```python
from build123d import *

# Parameters (mm, degrees)
SKETCH1_R           = 15
SKETCH1_R_2         = 3
BOSS_EXTRUDE1_DEPTH = 4
SKETCH2_R           = 15
SKETCH2_R_2         = 13
EXTRUDE_THIN1_DEPTH = 10
SKETCH3_R           = 25
SKETCH3_R_2         = 13
BOSS_EXTRUDE2_DEPTH = 4
CUT_EXTRUDE1_REACH  = 20
SKETCH4_R           = 1.75


with BuildPart() as part:
    # Sketch1 → Boss-Extrude1 (new body)
    with BuildSketch(Plane(origin=(0, 0, 0), x_dir=(1, 0, 0), z_dir=(0, 1, 0))):
        Circle(SKETCH1_R)
        Circle(SKETCH1_R_2, mode=Mode.SUBTRACT)
    extrude(amount=BOSS_EXTRUDE1_DEPTH)

    # Sketch2 → Extrude-Thin1 (add)
    with BuildSketch(Plane(origin=(0, 4, 0), x_dir=(1, 0, 0), z_dir=(0, 1, 0))):
        Circle(SKETCH2_R)
        Circle(SKETCH2_R_2, mode=Mode.SUBTRACT)
    extrude(amount=EXTRUDE_THIN1_DEPTH)

    # Sketch3 → Boss-Extrude2 (add)
    with BuildSketch(Plane(origin=(0, 14, 0), x_dir=(1, 0, 0), z_dir=(0, 1, 0))):
        Circle(SKETCH3_R)
        Circle(SKETCH3_R_2, mode=Mode.SUBTRACT)
    extrude(amount=BOSS_EXTRUDE2_DEPTH)

    # Sketch4 → Cut-Extrude1 (cut, up to next)
    with BuildSketch(Plane(origin=(0, 18, 0), x_dir=(1, 0, 0), z_dir=(0, 1, 0)), mode=Mode.PRIVATE) as cut_extrude1_sk1:
        with Locations((-17.320508076, 10)):
            Circle(SKETCH4_R)
    cut_extrude1_tool1 = extrude(cut_extrude1_sk1.sketch, amount=-CUT_EXTRUDE1_REACH, mode=Mode.PRIVATE) & part.part
    add(cut_extrude1_tool1.solids().sort_by_distance((-17.320508, 18, -10))[0], mode=Mode.SUBTRACT)
    # Sketch4 → Cut-Extrude1 (cut, up to next)
    with BuildSketch(Plane(origin=(0, 18, 0), x_dir=(1, 0, 0), z_dir=(0, 1, 0)), mode=Mode.PRIVATE) as cut_extrude1_sk2:
        with Locations((17.320508076, 10)):
            Circle(SKETCH4_R)
    cut_extrude1_tool2 = extrude(cut_extrude1_sk2.sketch, amount=-CUT_EXTRUDE1_REACH, mode=Mode.PRIVATE) & part.part
    add(cut_extrude1_tool2.solids().sort_by_distance((17.320508, 18, -10))[0], mode=Mode.SUBTRACT)
    # Sketch4 → Cut-Extrude1 (cut, up to next)
    with BuildSketch(Plane(origin=(0, 18, 0), x_dir=(1, 0, 0), z_dir=(0, 1, 0)), mode=Mode.PRIVATE) as cut_extrude1_sk3:
        with Locations((17.320508076, -10)):
            Circle(SKETCH4_R)
    cut_extrude1_tool3 = extrude(cut_extrude1_sk3.sketch, amount=-CUT_EXTRUDE1_REACH, mode=Mode.PRIVATE) & part.part
    add(cut_extrude1_tool3.solids().sort_by_distance((17.320508, 18, 10))[0], mode=Mode.SUBTRACT)
    # Sketch4 → Cut-Extrude1 (cut, up to next)
    with BuildSketch(Plane(origin=(0, 18, 0), x_dir=(1, 0, 0), z_dir=(0, 1, 0)), mode=Mode.PRIVATE) as cut_extrude1_sk4:
        with Locations((-17.320508076, -10)):
            Circle(SKETCH4_R)
    cut_extrude1_tool4 = extrude(cut_extrude1_sk4.sketch, amount=-CUT_EXTRUDE1_REACH, mode=Mode.PRIVATE) & part.part
    add(cut_extrude1_tool4.solids().sort_by_distance((-17.320508, 18, 10))[0], mode=Mode.SUBTRACT)


solid = part.part
```
Can you work these out from the model? Positions are in its coordinate system, mm. A direction names the side the tool comes from. Coordinates: 2 decimals unless noted, no trailing zeros. Order: outer loops, then holes, each group sorted by start corner. A loop starts at its lowest first (then second) coordinate and runs counter-clockwise, first axis right, second up. Notation, with made-up numbers: (-31.75, 21) -> (1.25, 21) arc R17 cw to (1.25, 38) -> close; hole circle Ø7 at (31, -33). An arc over 180 degrees is marked (long way). Write each question's results on one line, items separated by ' | '.
Item 1: I want a section at D-D, the plane x = 17. Write out the boundary of the cut face in (y, z), then the cut area to 3 significant figures.
Results are:
outline: (14, -18.33) -> (18, -18.33) -> (18, -11.72) -> (14, -11.72) -> close; (14, -8.28) -> (18, -8.28) -> (18, 8.28) -> (14, 8.28) -> close; (14, 11.72) -> (18, 11.72) -> (18, 18.33) -> (14, 18.33) -> close | area: 119 mm²
Item 2: I want a section at C-C, the plane y = 14.75. Write out the boundary of the cut face in (x, z), then the cut area to 3 significant figures.
Results are:
outline: circle Ø50 at (0, 0); hole circle Ø3.5 at (-17.32, -10); hole circle Ø3.5 at (-17.32, 10); hole circle Ø26 at (0, 0); hole circle Ø3.5 at (17.32, -10); hole circle Ø3.5 at (17.32, 10) | area: 1,390 mm²
Item 3: If I drill on line 1 along X through (y, z) = (15.45, 10); line 2 along Z through (x, y) = (0, 10.5); line 3 along X through (y, z) = (14.75, -9.5), over which ranges is the centre line in solid material (lowest first)?
Results are:
line 1: -22.91 to -19.07, -15.57 to -8.31, 8.31 to 15.57, 19.07 to 22.91 | line 2: -15 to -13, 13 to 15 | line 3: -23.12 to -19, -15.64 to -8.87, 8.87 to 15.64, 19 to 23.12
Item 4: I want a section at A-A, the plane x = 0. Write out the boundary of the cut face in (y, z), then the cut area to 3 significant figures.
Results are:
outline: (0, -15) -> (14, -15) -> (14, -25) -> (18, -25) -> (18, -13) -> (4, -13) -> (4, -3) -> (0, -3) -> close; (0, 3) -> (4, 3) -> (4, 13) -> (18, 13) -> (18, 25) -> (14, 25) -> (14, 15) -> (0, 15) -> close | area: 232 mm²
Item 5: If we mould it in two halves opening along Z, with no side actions, what happens to faces 1 (the face through (-3, 2, 0)), 2 (the face through (0, 0, -4)), 3 (the face through (23.846, 15.972, -7.509))? For each: +Z half, -Z half, draft (parallel to the pull), parting line (faces both ways), or undercut.
Results are:
face 1: undercut | face 2: draft | face 3: parting line
Item 6: I want a section at B-B, the plane z = 0. Write out the boundary of the cut face in (x, y).
Results are:
outline: (-25, 14) -> (-15, 14) -> (-15, 0) -> (-3, 0) -> (-3, 4) -> (-13, 4) -> (-13, 18) -> (-25, 18) -> close; (3, 0) -> (15, 0) -> (15, 14) -> (25, 14) -> (25, 18) -> (13, 18) -> (13, 4) -> (3, 4) -> close
Item 7: I'm going to push flat-ended pins straight in: pin 1 Ø5 at (x, y) = (-11.5, 7) entering from +Z; pin 2 Ø6 at (y, z) = (2.5, 6) entering from +X; pin 3 Ø3 at (x, z) = (17.32, 10) entering from +Y; pin 4 Ø4 at (y, z) = (4, 4) entering from -X. Where does each tip first touch, or does it pass through?
Results are:
pin 1: z = 12 | pin 2: x = 14.7 | pin 3: through | pin 4: x = -14.87
Item 8: Which directions (+Z, -Z, +X, -X, +Y, -Y) give clear straight access to the entire face, cutting with the end or side of a thin tool? Please do faces 4 (the face through (3, 4, 3)), 5 (the face through (-14.985, 6.902, -0.66)), 6 (the face through (18.99, 16.03, 9.47)).
Results are:
face 4: +Y | face 5: -Y | face 6: +Y, -Y
